Part model, mm, in its own coordinate system. A direction names the side the tool comes from. Give positions to 0.01 mm unless a question says otherwise; leave off trailing zeros. Order: outer loops, then holes, each group sorted by start corner. A loop starts at its lowest first (then second) coordinate and runs counter-clockwise, first axis right, second up. Notation, with made-up numbers: (9, 62.25) -> (48, 62.25) arc R28 ccw to (48, 98.25) -> close; hole circle Ø10 at (70.25, -4.75). An arc over 180 degrees is marked (long way). Write item = value, one per line. Start each with the question number.
Item 1: Band-saw the part on C-C on x = -117. Write the cut outline in (y, z).
Item 2: Tool access for faces 5 (the face through (145, -68.4, 13.9)), 6 (the face through (147.172, -79.774, 2.958)), 7 (the face through (110, -71, 3)), 8 (the face through (141, -68.4, 13.9)), 9 (the face through (143.03, -67.31, 12.17)): list every direction of +Z, -Z, +X, -X, +Y, -Y with a clear straight run to the whole face (end or side of a thin tool).
Item 3: Band-saw the part on A-A on x = -40. Write the cut outline in (y, z), plus the area to 3 significant figures.
Item 4: Band-saw the part on D-D on x = -77. Write the cut outline in (y, z), plus the area to 3 significant figures.
Item 5: Pull direction Y, two halves, no side cores. Call faces 1 (the face through (-2, -105, 3)), 2 (the face through (82, -65, 3)), 3 (the face through (-147.65, -78.51, 2.96)), 4 (the face through (-2, -70, 6)): +Y half, -Y half, draft (parallel to the pull), parting line (faces both ways), or undercut.
Item 6: Drill centre lines: line 1 along Y through (x, z) = (-110, 4.35); line 2 along Y through (x, z) = (-40, 1.9); line 3 along Z through (x, y) = (-31.5, -95). Where is each one in solid material? Low to high.
Item 7: Band-saw the part on B-B on y = -65. Write the cut outline in (x, z), plus the area to 3 significant figures.
Item 8: Flat gauge pins, fed straight in: P1, Ø8, axis at x = -92.5, y = -88.5, coming from the +Z side; P2, Ø2, axis at y = -60, z = 3.5, coming from the +X side; P3, Ø6, axis at y = -93, z = 4.5, coming from the +X side (3 decimals); P4, Ø3.5, axis at x = -96.21, y = -51.21, coming from the +Z side. Where does each tip first touch, or does it go through?
```python
from build123d import *

# Parameters (mm, degrees)
F0_R     = 3.25
F0_R_2   = 16
F1_DEPTH = 6
F2_W     = 4
F2_H     = 15
F3_DEPTH = 16
F4_R     = 3
F5_DEPTH = 25
F6_R     = 2
F7_DEPTH = 25


# Not quite as in the source:
# - ends of sketch curves that miss each other by under 0.0002 mm in the source are joined


with BuildPart() as f1:
    # F0 (on Top) → F1 (new body)
    with BuildSketch(Plane.XY):
        with BuildLine():
            ThreePointArc((110, -105), (147.4165738824, -79.1421355849), (136.4575130484, -34.9999999451))
            Line((136.4575130484, -34.9999999451), (75, -35))
            Line((75, -35), (-75, -35))
            Line((-75, -35), (-136.457514, -35))
            ThreePointArc((-136.457514, -35), (-147.4165737498, -79.1421359357), (-110, -105))
            Line((-110, -105), (-75, -105))
            Line((-75, -105), (75, -105))
            Line((75, -105), (110, -105))
        make_face()
        with Locations((40, -82)):
            Circle(F0_R, mode=Mode.SUBTRACT)
        with Locations((-110, -65)):
            Circle(F0_R_2, mode=Mode.SUBTRACT)
        with Locations((-40, -52)):
            Circle(F0_R, mode=Mode.SUBTRACT)
        with BuildLine():
            Line((88.000112, -59), (131.86291, -59.001567))
            ThreePointArc((131.86291, -59.001567), (137.9996084013, -64.9314505185), (132, -71))
            Line((132, -71), (88, -71))
            ThreePointArc((88, -71), (82.0000000003, -64.999944), (88.000112, -59))
        make_face(mode=Mode.SUBTRACT)
    extrude(amount=F1_DEPTH)

    # F2 (on face) → F3 (join)
    with BuildSketch(Plane.XY.offset(6)):
        with Locations((143, -64.9314505185)):
            Rectangle(F2_W, F2_H)
    extrude(amount=F3_DEPTH)

    # F4 (on face) → F5 (cut)
    with BuildSketch(Plane.YZ.offset(145)):
        with Locations((-64.9314505185, 14)):
            Circle(F4_R)
    extrude(amount=-F5_DEPTH, mode=Mode.SUBTRACT)

    # F6 (on face) → F7 (cut)
    with BuildSketch(Plane.XY.offset(6)):
        with Locations((-123.7885822331, -51.2114177669)):
            Circle(F6_R)
        with Locations((-96.2114177669, -51.2114177669)):
            Circle(F6_R)
        with Locations((-96.2114177669, -78.7885822331)):
            Circle(F6_R)
        with Locations((-123.7885822331, -78.7885822331)):
            Circle(F6_R)
    extrude(amount=-F7_DEPTH, mode=Mode.SUBTRACT)


solid = f1.part
```
Values found:
q1.outline = (-104.38, 0) -> (-79.39, 0) -> (-79.39, 6) -> (-104.38, 6) -> close; (-50.61, 0) -> (-35, 0) -> (-35, 6) -> (-50.61, 6) -> close
q2.face_5 = +Z, +X, +Y, -Y
q2.face_6 = +Z, -Z, +X
q2.face_7 = +Z, -Z
q2.face_8 = +Z, -X, +Y, -Y
q2.face_9 = +X, -X
q3.outline = (-105, 0) -> (-55.25, 0) -> (-55.25, 6) -> (-105, 6) -> close; (-48.75, 0) -> (-35, 0) -> (-35, 6) -> (-48.75, 6) -> close
q3.area = 381 mm^2
q4.outline = (-105, 0) -> (-35, 0) -> (-35, 6) -> (-105, 6) -> close
q4.area = 420 mm^2
q5.face_1 = -Y half
q5.face_2 = undercut
q5.face_3 = parting line
q5.face_4 = draft
q6.line_1 = -105 to -81, -49 to -35
q6.line_2 = -105 to -55.25, -48.75 to -35
q6.line_3 = 0 to 6
q7.outline = (-150, 0) -> (-126, 0) -> (-126, 6) -> (-150, 6) -> close; (-94, 0) -> (82, 0) -> (82, 6) -> (-94, 6) -> close; (138, 0) -> (150, 0) -> (150, 6) -> (145, 6) -> (145, 11) -> (141, 11) -> (141, 6) -> (138, 6) -> close; (141, 17) -> (145, 17) -> (145, 22) -> (141, 22) -> close
q7.area = 1,310 mm^2
q8.P1 = 6
q8.P2 = 149.8
q8.P3 = 141.225
q8.P4 = through
